```python
from build123d import *

# Parameters (mm, degrees)
SKETCH070_W      = 50
SKETCH070_H      = 76.5
EXTRUDE069_DEPTH = 3
SKETCH069_W      = 50
SKETCH069_H      = 80
SKETCH069_R      = 2.6
SKETCH069_W_2    = 35
SKETCH069_H_2    = 54
EXTRUDE068_DEPTH = 9
SKETCH061_R      = 1.85
EXTRUDE060_DEPTH = 15
SKETCH076_R      = 2.85
EXTRUDE075_DEPTH = 10
EXTRUDE059_DEPTH = 15
EXTRUDE058_DEPTH = 104
ARRAY018_COUNT   = 2


with BuildPart() as extrude069:
    # Sketch070 → Extrude069 (new body)
    with BuildSketch(Plane.XY):
        Rectangle(SKETCH070_W, SKETCH070_H)
    extrude(amount=EXTRUDE069_DEPTH)


with BuildPart() as extrude069_1:
    # Extrude069 placement: moved
    add(extrude069.part.moved(Location((0, 0, -9))))


with BuildPart() as cut040:
    # Sketch069 → Extrude068 (new body)
    with BuildSketch(Plane.XY):
        Rectangle(SKETCH069_W, SKETCH069_H)
        with Locations((0, 32.5)):
            Circle(SKETCH069_R, mode=Mode.SUBTRACT)
        with Locations((0, -32.5)):
            Circle(SKETCH069_R, mode=Mode.SUBTRACT)
        Rectangle(SKETCH069_W_2, SKETCH069_H_2, mode=Mode.SUBTRACT)
    extrude(amount=-EXTRUDE068_DEPTH)

    # Cut040: cut Extrude069
    add(extrude069_1.part, mode=Mode.SUBTRACT)


with BuildPart() as extrude060:
    # Sketch061 → Extrude060 (new body)
    with BuildSketch(Plane.XY):
        with Locations((-37.5, -7)):
            Circle(SKETCH061_R)
        with Locations((0, -7)):
            Circle(SKETCH061_R)
        with Locations((37.5, -7)):
            Circle(SKETCH061_R)
    extrude(amount=-EXTRUDE060_DEPTH)


with BuildPart() as fusion034004041012:
    # Sketch076 → Extrude075 (new body)
    with BuildSketch(Plane.XY):
        with Locations((-37.5, -7)):
            Circle(SKETCH076_R)
        with Locations((0, -7)):
            Circle(SKETCH076_R)
        with Locations((37.5, -7)):
            Circle(SKETCH076_R)
    extrude(amount=-EXTRUDE075_DEPTH)


with BuildPart() as fusion034004041012_1:
    # Extrude075 placement: moved
    add(fusion034004041012.part.moved(Location((0, 0, -5))))

    # Fusion034004041012: union Extrude060
    add(extrude060.part)


with BuildPart() as extrude059:
    # Sketch060 → Extrude059 (new body)
    with BuildSketch(Plane.XZ):
        with BuildLine():
            ThreePointArc((-25, -7.5), (-28, -10.5), (-25, -13.5))
            Line((-25, -13.5), (-15, -13.5))
            ThreePointArc((-15, -13.5), (-12, -10.5), (-15, -7.5))
            Line((-25, -7.5), (-15, -7.5))
        make_face()
        with BuildLine():
            ThreePointArc((-5, -7.5), (-8, -10.5), (-5, -13.5))
            Line((-5, -13.5), (5, -13.5))
            ThreePointArc((5, -13.5), (8, -10.5), (5, -7.5))
            Line((-5, -7.5), (5, -7.5))
        make_face()
        with BuildLine():
            ThreePointArc((15, -7.5), (12, -10.5), (15, -13.5))
            Line((15, -13.5), (25, -13.5))
            ThreePointArc((25, -13.5), (28, -10.5), (25, -7.5))
            Line((15, -7.5), (25, -7.5))
        make_face()
        with BuildLine():
            ThreePointArc((35, -7.5), (32, -10.5), (35, -13.5))
            Line((35, -13.5), (45, -13.5))
            ThreePointArc((45, -13.5), (48, -10.5), (45, -7.5))
            Line((35, -7.5), (45, -7.5))
        make_face()
        with BuildLine():
            ThreePointArc((-45, -7.5), (-48, -10.5), (-45, -13.5))
            Line((-45, -13.5), (-35, -13.5))
            ThreePointArc((-35, -13.5), (-32, -10.5), (-35, -7.5))
            Line((-45, -7.5), (-35, -7.5))
        make_face()
    extrude(amount=EXTRUDE059_DEPTH)


with BuildPart() as extrude059_1:
    # Extrude059 placement: moved
    add(extrude059.part.moved(Location((0, -7, -2))))


with BuildPart() as landinggearfusion030:
    # Sketch059 → Extrude058 (new body)
    with BuildSketch(Plane.YZ):
        Polygon((0, 0), (-12, 0), (-22.392305, -18), (-12.392305, -18), (-7.196152, -9), (0, -9), align=None)
    extrude(amount=EXTRUDE058_DEPTH)


with BuildPart() as landinggearfusion030_1:
    # Extrude058 placement: moved
    add(landinggearfusion030.part.moved(Location((-52, 0, 0))))

    # Cut033: cut Extrude059
    add(extrude059_1.part, mode=Mode.SUBTRACT)

    # Cut041: cut Fusion034004041012
    add(fusion034004041012_1.part, mode=Mode.SUBTRACT)


with BuildPart() as landinggearfusion030_2:
    # Cut041 placement: moved
    add(landinggearfusion030_1.part.moved(Location((0, -39.5, 0))))

    # Array018: LandingGearFusion030 ×2 about axis
    array018_axis = Axis((0, 0, 0), (0, 0, 1))


with BuildPart() as landinggearfusion030_3:
    add(landinggearfusion030_2.part)
    for i in range(1, ARRAY018_COUNT):
        add(landinggearfusion030_2.part.rotate(array018_axis, i * 360 / ARRAY018_COUNT))

    # Fusion030: union Cut040
    add(cut040.part)


with BuildPart() as landinggearfusion030_4:
    # Fusion030 placement: moved
    add(landinggearfusion030_3.part.moved(Location((0, 0, -70))))


solid = landinggearfusion030_4.part
```
Build history of the part. All positions in model axes, mm. A direction names the side the tool comes from. Give positions to 0.01 mm unless a question says otherwise; leave off trailing zeros. Order: outer loops, then holes, each group sorted by start corner. A loop starts at its lowest first (then second) coordinate and runs counter-clockwise, first axis right, second up. Notation, with made-up numbers: M 49.5,36 L 70.5,36 A4 cw 70.5,43 Z; hole C 10,-37 d4. An arc over 180 degrees is marked long. Write item = value, one per line. Start each with the question number.
(1) Pin check, flat tips, straight feed: pin 1 Ø3 at (x, y) = (-21.5, 57) entering from +Z; pin 2 Ø8 at (x, z) = (17.5, -74) entering from +Y; pin 3 Ø6 at (y, z) = (15, -74) entering from +X. Stop position of each tip, or through.
(2) Probe L1, parallel to X at y = -46.5, z = -75.95; L2, parallel to Y at x = 1, z = -76.75; L3, parallel to Y at x = 37.5, z = -73.85. List the from-to ranges inside material, lowest first. Write a range as [from, to].
(3) Two-plate mould, pull along X, no slides. Class faces 5 (the flat face through (40, -52, -79.5)), 6 (the flat face through (0.73, 51.06, -86.56)): released by +X, released by -X, zero draft, split by the parting line, or undercut.
(4) Slice it at A-A on x = 37.5. State how many separate pieces and enclosed holes the cut face has, plus the area to 3 significant figures.
(5) Slice it at B-B on x = -42. Write the cut outline in (y, z).
(6) Which spindle directions (+Z, -Z, +X, -X, +Y, -Y) get a long thin tool onto all of the face, cutting with end or side? Do faces 1 (the flat face through (-38, 39.5, -75)), 2 (the flat face through (-0.73, -51.06, -86.56)), 3 (the cylindrical face through (-0.62, -49.28, -77.22)), 4 (the flat face through (0, 27, -73)). Say none if no direction does.
Responses:
q1.pin_1 = -76.93
q1.pin_2 = 56.12
q1.pin_3 = 25
q2.L1 = [-52, -40.35], [-34.65, -2.85], [2.85, 34.65], [40.35, 52]
q2.L2 = [-55.4, -49.17], [-43.83, -38.25], [38.25, 43.83], [49.17, 55.4]
q2.L3 = [-53.72, -48.35], [-44.65, -39.5], [39.5, 44.65], [48.35, 53.72]
q3.face_5 = undercut
q3.face_6 = zero draft
q4.separate_pieces = 6
q4.enclosed_holes = 0
q4.area = 238 mm2
q5.outline = M -61.89,-88 L -51.89,-88 L -50.45,-85.5 L -60.45,-85.5 Z; M -56.98,-79.5 L -46.98,-79.5 L -46.7,-79 L -39.5,-79 L -39.5,-70 L -51.5,-70 Z; M 39.5,-79 L 46.7,-79 L 46.98,-79.5 L 56.98,-79.5 L 51.5,-70 L 39.5,-70 Z; M 50.45,-85.5 L 51.89,-88 L 61.89,-88 L 60.45,-85.5 Z
q6.face_1 = +Z, -Z, -X
q6.face_2 = -Z, +X, -X
q6.face_3 = -Z
q6.face_4 = +Z, -Z
